Here's how the part is built. I have some questions about the finished solid (model axes, mm). A direction names the side the tool comes from. Round coordinates to 2 decimals unless told otherwise and drop trailing zeros. Order: outer loops, then holes, each group sorted by start corner. A loop starts at its lowest first (then second) coordinate and runs counter-clockwise, first axis right, second up. Notation, with made-up numbers: (1, 51.5) - (7, 51.5) arc R15 cw to (7, 64.5) - close; hole circle Ø5 at (21, -29.75). An arc over 180 degrees is marked (long way). One line per item, written item: value.
from build123d import *

# Parameters (mm, degrees)
F0_R     = 38.1
F1_DEPTH = 50.8
F2_R     = 22.86
F3_DEPTH = 9.398
F4_R     = 22.86
F5_DEPTH = 9.398
F6_R     = 4.7625
F7_DEPTH = 101.601
F8_R     = 1.6383
F9_DEPTH = 92.203


with BuildPart() as f1:
    # F0 (on Right) → F1 (new body, symmetric)
    with BuildSketch(Plane.YZ):
        Circle(F0_R)
    extrude(amount=F1_DEPTH, both=True)

    # F2 (on face) → F3 (cut)
    with BuildSketch(Plane(origin=(-50.8, 0, 0), x_dir=(0, -1, 0), z_dir=(-1, 0, 0))):
        Circle(F2_R)
    extrude(amount=-F3_DEPTH, mode=Mode.SUBTRACT)

    # F4 (on face) → F5 (cut)
    with BuildSketch(Plane.YZ.offset(50.8)):
        Circle(F4_R)
    extrude(amount=-F5_DEPTH, mode=Mode.SUBTRACT)

    # F6 (on face) → F7 (cut, through all)
    with BuildSketch(Plane(origin=(-50.8, 0, 0), x_dir=(0, -1, 0), z_dir=(-1, 0, 0))):
        Circle(F6_R)
    extrude(amount=-F7_DEPTH, mode=Mode.SUBTRACT)

    # F8 (on face) → F9 (cut, through all)
    with BuildSketch(Plane(origin=(-41.402, 0, 0), x_dir=(0, -1, 0), z_dir=(-1, 0, 0))):
        with Locations((0, 14.6812)):
            Circle(F8_R)
        with Locations((12.714292, 7.3406)):
            Circle(F8_R)
        with Locations((12.714292, -7.3406)):
            Circle(F8_R)
        with Locations((0, -14.6812)):
            Circle(F8_R)
        with Locations((-12.714292, -7.3406)):
            Circle(F8_R)
        with Locations((-12.714292, 7.3406)):
            Circle(F8_R)
    extrude(amount=-F9_DEPTH, mode=Mode.SUBTRACT)


solid = f1.part
Q1. If we section it at B-B, the plane y = 0: Please give me the cut outline in (x, z), then the cut area to 3 significant figures.
Results list:
outline: (-50.8, -38.1) - (50.8, -38.1) - (50.8, -22.86) - (41.4, -22.86) - (41.4, -16.32) - (-41.4, -16.32) - (-41.4, -22.86) - (-50.8, -22.86) - close; (-50.8, 22.86) - (-41.4, 22.86) - (-41.4, 16.32) - (41.4, 16.32) - (41.4, 22.86) - (50.8, 22.86) - (50.8, 38.1) - (-50.8, 38.1) - close; (-41.4, -13.04) - (41.4, -13.04) - (41.4, -4.76) - (-41.4, -4.76) - close; (-41.4, 4.76) - (41.4, 4.76) - (41.4, 13.04) - (-41.4, 13.04) - close
area: 5,550 mm²
Q2. If we section it at A-A, the plane z = 0: Please give me the cut outline in (x, y).
Results list:
outline: (-50.8, -38.1) - (50.8, -38.1) - (50.8, -22.86) - (41.4, -22.86) - (41.4, -4.76) - (-41.4, -4.76) - (-41.4, -22.86) - (-50.8, -22.86) - close; (-50.8, 22.86) - (-41.4, 22.86) - (-41.4, 4.76) - (41.4, 4.76) - (41.4, 22.86) - (50.8, 22.86) - (50.8, 38.1) - (-50.8, 38.1) - close
Q3. Will these pins go through, and if not, where does the flat tip stop? pin 1 (13.5 mm diameter, centred on y = 1.5, z = -3.5, fed in from +X); pin 2 (8 mm diameter, centred on x = -35, y = 26, fed in from -Z); pin 3 (4 mm diameter, centred on x = 6, y = -21.5, fed in from +Z); pin 4 (2.5 mm diameter, centred on y = 0, z = -14.68, fed in from +X).
Results list:
pin 1: x = 41.4
pin 2: z = -31.11
pin 3: z = 32.73
pin 4: through
Q4. If we section it at D-D, the plane z = -20.5: Please give me the cut outline in (x, y).
Results list:
outline: (-50.8, -32.11) - (50.8, -32.11) - (50.8, -10.12) - (41.4, -10.12) - (41.4, 10.12) - (50.8, 10.12) - (50.8, 32.11) - (-50.8, 32.11) - (-50.8, 10.12) - (-41.4, 10.12) - (-41.4, -10.12) - (-50.8, -10.12) - close
Q5. We'd pull the mould along Y, two halves only. Please class faces 4 (the cylindrical face through (0.711, -30.235, -23.183)), 5 (the flat face through (-50.8, 16.4, -16.4)), 6 (the cylindrical face through (-0.58, -12.36, 5.74)), 7 (the cylindrical face through (-0.58, -0.756, -16.135)): released by +Y, released by -Y, zero draft, split by the parting line, or undercut.
Results list:
face 4: split by the parting line
face 5: zero draft
face 6: undercut
face 7: undercut
Q6. If we section it at C-C, the plane x = 33: Please give me the cut outline in (y, z) (1 decimal).
Results list:
outline: circle Ø76.2 at (0, 0); hole circle Ø3.3 at (-12.7, -7.3); hole circle Ø3.3 at (-12.7, 7.3); hole circle Ø9.5 at (0, 0); hole circle Ø3.3 at (0, -14.7); hole circle Ø3.3 at (0, 14.7); hole circle Ø3.3 at (12.7, -7.3); hole circle Ø3.3 at (12.7, 7.3)
Q7. Which directions (+Z, -Z, +X, -X, +Y, -Y) give clear straight access to the entire face, cutting with the end or side of a thin tool? Please do faces 1 (the cylindrical face through (46.167, 21.804, 6.867)), 2 (the cylindrical face through (-46.167, -21.804, 6.867)), 3 (the cylindrical face through (-0.58, 3.78, -2.9)).
Results list:
face 1: +X
face 2: -X
face 3: +X, -X
Q8. If I drill on line 1 along Z through (x, y) = (-21, 0); line 2 along Y through (x, z) = (12.5, 0.5); line 3 along Z through (x, y) = (47, 0), over which ranges is the centre line in solid material (lowest first)?
Results list:
line 1: -38.1 to -16.32, -13.04 to -4.76, 4.76 to 13.04, 16.32 to 38.1
line 2: -38.1 to -4.74, 4.74 to 38.1
line 3: -38.1 to -22.86, 22.86 to 38.1
